from build123d import *

# Parameters (mm, degrees)
SKETCH1_R           = 150
SKETCH1_R_2         = 138
BOSS_EXTRUDE1_DEPTH = 40
FILLET1_R           = 3
BOSS_EXTRUDE2_DEPTH = 12.5
BOSS_EXTRUDE3_DEPTH = 5.5
SKETCH6_R           = 6.730891085
BOSS_EXTRUDE4_DEPTH = 3
BOSS_EXTRUDE4_TAPER = 30
SKETCH8_R           = 7.5
CUT_EXTRUDE1_DEPTH  = 229.714341483


with BuildPart() as part:
    # Sketch1 → Boss-Extrude1 (new, symmetric)
    with BuildSketch(Plane.XY):
        Circle(SKETCH1_R)
        Circle(SKETCH1_R_2, mode=Mode.SUBTRACT)
    extrude(amount=BOSS_EXTRUDE1_DEPTH, both=True)

    # Fillet1
    fillet1_edges = [part.edges().sort_by_distance(p)[0] for p in [
        (-150, 0, -40),
        (-150, 0, 40),
    ]]
    fillet(fillet1_edges, radius=FILLET1_R)



with BuildPart() as body_2:
    # Sketch2 → Revolve1 (revolve)
    with BuildSketch(Plane(origin=(0, 0, 0), x_dir=(1, 0, 0), z_dir=(0, 1, 0)), mode=Mode.PRIVATE) as revolve1_sk:
        Polygon((0, 42), (0, -42), (-38, -42), (-38, -43.5), (-44, -43.5), (-50.171444325, -8.5), (-120.445700108, -8.5), (-126, -40), (-138, -40), (-138, 40), (-126, 40), (-120.445700108, 8.5), (-50.171444325, 8.5), (-44, 43.5), (-38, 43.5), (-38, 42), align=None)
    revolve(revolve1_sk.sketch.rotate(Axis((0, 0, 0), (0, 0, -1)), 180), axis=Axis((0, 0, 0), (0, 0, -1)))


with BuildPart() as part_1:
    add(part.part)

    add(body_2.part)  # Boss-Extrude2 merges body 2
    # Sketch4 → Boss-Extrude2 (add, symmetric)
    with BuildSketch(Plane(origin=(0, 0, 0), x_dir=(1, 0, 0), z_dir=(0, 1, 0))):
        Polygon((-36.665910449, 28.5), (-36.665910449, 8.5), (-71.665910449, 8.5), (-71.665910449, 11.5), (-39.665910449, 28.5), align=None)
    extrude(amount=BOSS_EXTRUDE2_DEPTH, both=True)

    # Sketch5 → Boss-Extrude3 (add)
    with BuildSketch(Plane(origin=(-20.538802833, 0, -38.661275921), x_dir=(-0.8831157194574106, 0, 0.46915522596174936), z_dir=(-0.4691552259617493, 0, -0.8831157194574105))):
        Polygon((49.851566833, 3.4173178), (43.40179394, 7.754016548), (36.42121621, 4.336698747), (35.890411372, -3.4173178), (42.340184265, -7.754016548), (49.320761995, -4.336698747), align=None)
    extrude(amount=BOSS_EXTRUDE3_DEPTH)

    # Sketch6 → Boss-Extrude4 (add)
    with BuildSketch(Plane(origin=(-23.119156576, 0, -43.518412378), x_dir=(-0.8831157194574103, 0, 0.4691552259617501), z_dir=(-0.4691552259617501, 0, -0.8831157194574103))):
        with Locations((42.870989102, 0)):
            Circle(SKETCH6_R)
    extrude(amount=BOSS_EXTRUDE4_DEPTH, taper=BOSS_EXTRUDE4_TAPER)

    # Sketch7 → Revolve3 (revolve)
    with BuildSketch(Plane(origin=(0, 0, 0), x_dir=(1, 0, 0), z_dir=(0, 1, 0))):
        with BuildLine():
            ThreePointArc((-66.505399661, 33.471675934), (-60.781448215, 33.38765917), (-57.972112211, 28.399842997))
            Line((-57.972112211, 28.399842997), (-62.386666639, 26.054610957))
            Line((-62.386666639, 26.054610957), (-66.505399661, 33.471675934))
        make_face()
    revolve(axis=Axis((-62.386666639, 0, -26.054610957), (-0.4854755142964054, 0, -0.8742502645230602)))

    # Sketch8 → Cut-Extrude1 (cut, through all)
    with BuildSketch(Plane(origin=(0, 0, -42), x_dir=(-1, 0, 0), z_dir=(0, 0, -1))):
        Circle(SKETCH8_R)
    extrude(amount=-CUT_EXTRUDE1_DEPTH, mode=Mode.SUBTRACT)


solid = part_1.part
Source: CAD feature listing. Evaluate the final solid. Frame: model axes, mm. A direction names the side the tool comes from. Round coordinates to 2 decimals unless told otherwise and drop trailing zeros. Loops run counter-clockwise (first coordinate to the right, second up) from the corner with the lowest first, then second, coordinate; pieces in that order, holes last.
Q1. Ray query, line 1 (Y direction, x = 0, z = 43.05); line 2 (Y direction, x = 0, z = 3); line 3 (Y direction, x = 0, z = 20.5). Return the intervals inside material, ascending.
Q2. First-contact query: P1, Ø8.5, axis at x = -54.5, z = -21, coming from the +Y side; P2, Ø3, axis at x = 57, y = 103.5, coming from the +Z side; P3, Ø12, axis at x = 96, z = 28, coming from the -Y side. Flat tips, straight axial feed; report the tip coordinate or a pass-through.
Q3. Section A-A, the plane z = 12.5. Return loops of the section in (x, y).
Q4. Access query for faces 1 (the face through (-62.24, -6.07, -19.58)), 2 (the face through (1, 8, 42)), 3 (the face through (-57.1, 6.07, -22.31)), 4 (the face through (36, 13, 43.5)). Directions: +Z, -Z, +X, -X, +Y, -Y. A direction counts if a zero-diameter tool reaches every point of the face in a straight line with its end or side. Return the directions, or none.
Q5. Section C-C, the plane z = 31. Return loops of the section in (x, y), plus the area to 3 significant figures.
Q6. Mould query, pull axis X, two halves, no side actions, for faces 5 (the face through (-19.527, 148.724, 0.518)), 6 (the face through (-108, -66, 40)), 7 (the face through (115.215, -36.283, 10.47)). Classes: pulls with the +X half, pulls with the -X half, needs draft (parallel to the pull), parting line crosses it, or undercut.
Q7. Section B-B, the plane z = -4. Return loops of the section in (x, y).
Solutions:
1. line 1: y = -44.08 to -38, 38 to 44.08
1. line 2: y = -150 to -7.5, 7.5 to 150
1. line 3: y = -150 to -122.56, -48.06 to -7.5, 7.5 to 48.06, 122.56 to 150
2. P1: stops at y = 141.33
2. P2: stops at z = 8.5
2. P3: stops at y = -120
3. outline: circle Ø300 at (0, 0); circle Ø98.93 at (0, 0); hole circle Ø242.3 at (0, 0); hole circle Ø15 at (0, 0)
4. face 1: none
4. face 2: +Z
4. face 3: -Z
4. face 4: +Z, +X, -X, +Y, -Y
5. outline: circle Ø300 at (0, 0); circle Ø92.41 at (0, 0); hole circle Ø248.83 at (0, 0); hole circle Ø15 at (0, 0)
5. area: 28,600 mm2
6. face 5: parting line crosses it
6. face 6: needs draft
6. face 7: undercut
7. outline: circle Ø300 at (0, 0); hole circle Ø15 at (0, 0)
